Geometry: see drawing. Coordinates: mm, zero at the bounding-box minimum. Round coordinates to 2 decimals unless told otherwise and drop trailing zeros. Order: outer loops, then holes, each group sorted by start corner. A loop starts at its lowest first (then second) coordinate and runs counter-clockwise, first axis right, second up. Notation, with made-up numbers: (10.5, 70.25) -> (17.5, 70.25) arc R14 ccw to (17.5, 86.25) -> close; hole circle Ø1 at (32, 81). An arc over 180 degrees is marked (long way). Answer as CSV lines item,"result". Start each with the question number.
(1) Section query C-C (y = 17). Output: boundary loops of the cut face in (x, z).
(2) Section query A-A (x = 10). Output: boundary loops of the cut face in (y, z).
(3) Section query B-B (z = 0.8). Count the separate pieces of the cut face and the enclosed holes in it, plus the area to 3 significant figures.
(4) Section query D-D (x = 7.5). Output: boundary loops of the cut face in (y, z) (1 decimal).
(5) Pull-direction query (X, two-part tool) for the marked faces 1, 2 and 3; classes: +X half, -X half, draft (parallel to the pull), parting line (faces both ways), or undercut.
(6) Line query: line 1 along Y through (x, z) = (14.75, 1.95) (1 decimal); line 2 along Y through (x, z) = (5, 2.7) (1 decimal); line 3 along X through (y, z) = (22.5, 1.2) (1 decimal). Output: solid intervals per line, ascending. Write a range as from..to.
(7) Contact query for a flat-ended pin moving along its axis: P1, Ø4, axis at x = 10.5, y = 6.13, coming from the -Z side. Output: stop coordinate, or through.
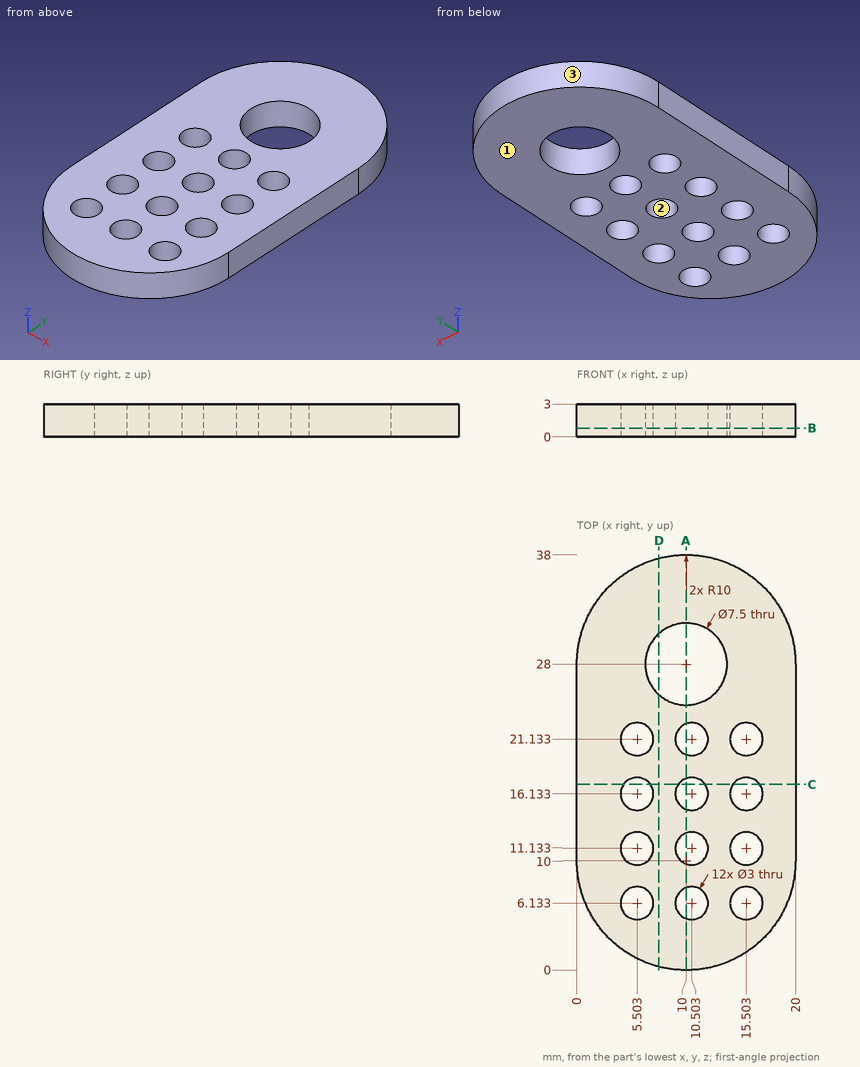
Answer block:
1,outline,"(0, 0) -> (4.28, 0) -> (4.28, 3) -> (0, 3) -> close; (6.73, 0) -> (9.28, 0) -> (9.28, 3) -> (6.73, 3) -> close; (11.73, 0) -> (14.28, 0) -> (14.28, 3) -> (11.73, 3) -> close; (16.73, 0) -> (20, 0) -> (20, 3) -> (16.73, 3) -> close"
2,outline,"(0, 0) -> (4.72, 0) -> (4.72, 3) -> (0, 3) -> close; (7.55, 0) -> (9.72, 0) -> (9.72, 3) -> (7.55, 3) -> close; (12.55, 0) -> (14.72, 0) -> (14.72, 3) -> (12.55, 3) -> close; (17.55, 0) -> (19.72, 0) -> (19.72, 3) -> (17.55, 3) -> close; (22.55, 0) -> (24.25, 0) -> (24.25, 3) -> (22.55, 3) -> close; (31.75, 0) -> (38, 0) -> (38, 3) -> (31.75, 3) -> close"
3,separate pieces,"1"
3,enclosed holes,"13"
3,area,"545 mm2"
4,outline,"(0.3, 0) -> (25.2, 0) -> (25.2, 3) -> (0.3, 3) -> close; (30.8, 0) -> (37.7, 0) -> (37.7, 3) -> (30.8, 3) -> close"
5,face 1,"draft"
5,face 2,"undercut"
5,face 3,"parting line"
6,line 1,"1.2..4.8, 7.4..9.8, 12.4..14.8, 17.4..19.8, 22.4..36.8"
6,line 2,"1.3..4.7, 7.5..9.7, 12.5..14.7, 17.5..19.7, 22.5..36.7"
6,line 3,"0..4.9, 6.1..9.9, 11.1..14.9, 16.1..20"
7,P1,"z = 0"
